from build123d import *

# Parameters (mm, degrees)
SKETCH1_W                    = 10
SKETCH1_H                    = 30
BOSS_EXTRUDE1_DEPTH          = 33.2
SKETCH2_R                    = 4.205
CUT_EXTRUDE1_DEPTH           = 38.778830051
CUT_EXTRUDE2_DEPTH           = 3.12
SKETCH4_W                    = 60
SKETCH4_H                    = 5
BOSS_EXTRUDE2_DEPTH          = 10
FILLET1_R                    = 5
BOSS_EXTRUDE3_START          = 5
BOSS_EXTRUDE3_DEPTH          = 5
CUT_EXTRUDE_THIN1_DEPTH      = 48.19364364
CUT_EXTRUDE_THIN1_DEPTH_BACK = 1.5
CUT_EXTRUDE_THIN2_DEPTH      = 48.19364364
CUT_EXTRUDE_THIN2_DEPTH_BACK = 1.5


with BuildPart() as part:
    # Sketch1 → Boss-Extrude1 (new body)
    with BuildSketch(Plane(origin=(0, 0, 0), x_dir=(1, 0, 0), z_dir=(0, 1, 0))):
        Rectangle(SKETCH1_W, SKETCH1_H)
    extrude(amount=BOSS_EXTRUDE1_DEPTH)

    # Sketch2 → Cut-Extrude1 (cut, through all)
    with BuildSketch(Plane.ZY.offset(5)):
        with Locations((0, 33.2)):
            Circle(SKETCH2_R)
    extrude(amount=-CUT_EXTRUDE1_DEPTH, mode=Mode.SUBTRACT)

    # Sketch3 → Cut-Extrude2 (cut)
    with BuildSketch(Plane(origin=(0, 33.2, 0), x_dir=(1, 0, 0), z_dir=(0, 1, 0))):
        Polygon((2.020725942, 6.5), (4.041451884, 10), (2.020725942, 13.5), (-2.020725942, 13.5), (-4.041451884, 10), (-2.020725942, 6.5), align=None)
    cut_extrude2 = extrude(amount=-CUT_EXTRUDE2_DEPTH, mode=Mode.SUBTRACT)

    # Mirror1: Cut-Extrude2 across plane
    add(cut_extrude2.mirror(Plane.XY), mode=Mode.SUBTRACT)

    # Sketch4 → Boss-Extrude2 (add)
    with BuildSketch(Plane(origin=(5, 0, 0), x_dir=(0, 0, -1), z_dir=(1, 0, 0))):
        with Locations((0, 2.5)):
            Rectangle(SKETCH4_W, SKETCH4_H)
    extrude(amount=-BOSS_EXTRUDE2_DEPTH)

    # Fillet1
    fillet1_edges = [part.edges().sort_by_distance(p)[0] for p in [
        (0, 5, -15),
        (0, 5, 15),
    ]]
    fillet(fillet1_edges, radius=FILLET1_R)

    # Sketch5 → Boss-Extrude3 (add)
    with BuildSketch(Plane.ZY.offset(5).offset(BOSS_EXTRUDE3_START)):
        with BuildLine():
            Line((-10, 33.2), (-4.205, 33.2))
            ThreePointArc((-4.205, 33.2), (0, 28.995), (4.205, 33.2))
            Line((4.205, 33.2), (10, 33.2))
            ThreePointArc((10, 33.2), (0, 23.2), (-10, 33.2))
        make_face()
    extrude(amount=-BOSS_EXTRUDE3_DEPTH)

    # Sketch6 → Cut-Extrude-Thin1 (cut, two sides: drawn at the far end of the back side and taken through both)
    with BuildSketch(Plane.ZY.offset(10).offset(-CUT_EXTRUDE_THIN1_DEPTH_BACK)):
        Polygon((-0.649519053, 32.825), (4.350480947, 24.164745962), (5.649519053, 24.914745962), (0.649519053, 33.575), align=None)
    extrude(amount=CUT_EXTRUDE_THIN1_DEPTH + CUT_EXTRUDE_THIN1_DEPTH_BACK, mode=Mode.SUBTRACT)

    # Sketch7 → Cut-Extrude-Thin2 (cut, two sides: drawn at the far end of the back side and taken through both)
    with BuildSketch(Plane.ZY.offset(10).offset(-CUT_EXTRUDE_THIN2_DEPTH_BACK)):
        Polygon((-0.649519053, 33.575), (-5.649519053, 24.914745962), (-4.350480947, 24.164745962), (0.649519053, 32.825), align=None)
    extrude(amount=CUT_EXTRUDE_THIN2_DEPTH + CUT_EXTRUDE_THIN2_DEPTH_BACK, mode=Mode.SUBTRACT)


solid = part.part
Input: part model. Units: mm. Frame: model coordinates. A direction names the side the tool comes from. Round coordinates to 2 decimals unless told otherwise and drop trailing zeros. Write each loop counter-clockwise with the first axis right and the second up, starting at its lowest first coordinate (ties: lowest second). Pieces come first, ordered by that corner, then holes.
1) Draft query along Y for faces 1 (the flat face through (-9.24, 26.75, 2.86)), 2 (the flat face through (0, 5, 25)), 3 (the cylindrical face through (-7.5, 23.2, 0.2)). Return one class per face: pulls with the +Y half, pulls with the -Y half, needs draft (parallel to the pull), parting line crosses it, or undercut.
2) Cut plane C-C (y = 3). Return the cut outline in (x, z).
3) Contact query for flat-ended pins moving along their axis: P1, Ø1.6, axis at x = -0.5, y = 31, coming from the +Z side; P2, Ø1.5, axis at x = -2.5, y = 7.5, coming from the -Z side; P3, Ø2, axis at x = 2, z = 9.5, coming from the +Y side. Output: stop coordinate, or through.
4) Reachability of faces 4 (the flat face through (-3, 33.2, 7)), 5 (the flat face through (3.045, 31.662, -11.726)), 6 (the flat face through (-9.24, 27.43, 4.197)), 7 (the flat face through (0, 21, 15)), 8 (the flat face through (0, 21, -15)) from +Z, -Z, +X, -X, +Y, -Y: full face, straight path, thin tool, end or side. Return the list, or none.
5) Ray query, L1, parallel to X at y = 22.5, z = -9; L2, parallel to Z at x = -4, y = 15; L3, parallel to Z at x = 2.5, y = 30.5. Return the intervals inside material, ascending.
6) Cut plane D-D (x = -6.5). Return the cut outline in (y, z) (3 decimals).
7) Cut plane A-A (x = -0.5). Return the cut outline in (y, z) (3 decimals), then the cut area to 3 significant figures.
8) Cut plane B-B (z = 0). Return the cut outline in (x, y) (3 decimals).
Geometry says:
1. face 1: undercut
1. face 2: pulls with the +Y half
1. face 3: pulls with the -Y half
2. outline: (-5, -30) - (5, -30) - (5, 30) - (-5, 30) - close
3. P1: stops at z = 15
3. P2: stops at z = -16.2
3. P3: stops at y = 30.08
4. face 4: +Z, -Z, +X, -X, +Y
4. face 5: +Y
4. face 6: -X
4. face 7: +Z, +X, -X, +Y
4. face 8: -Z, +X, -X, +Y
5. L1: x = -5 to 5
5. L2: z = -15 to 15
5. L3: z = -15 to -12.67, -7.33 to -3.22, 3.22 to 7.33, 12.67 to 15
6. outline: (33.2, -10) - (33.2, -4.205) arc R4.205 cw to (33.2, 4.205) - (33.2, 10) arc R10 ccw to start
7. outline: (0, -30) - (5, -30) - (5, -20) arc R5 cw to (10, -15) - (33.2, -15) - (33.2, -13.5) - (30.08, -13.5) - (30.08, -6.5) - (33.2, -6.5) - (33.2, -4.205) arc R4.205 cw to (33.2, 4.205) - (33.2, 6.5) - (30.08, 6.5) - (30.08, 13.5) - (33.2, 13.5) - (33.2, 15) - (10, 15) arc R5 cw to (5, 20) - (5, 30) - (0, 30) - close
7. area: 1,090 mm2
8. outline: (-10, 23.2) - (-5, 23.2) - (-5, 0) - (5, 0) - (5, 28.995) - (-10, 28.995) - close
